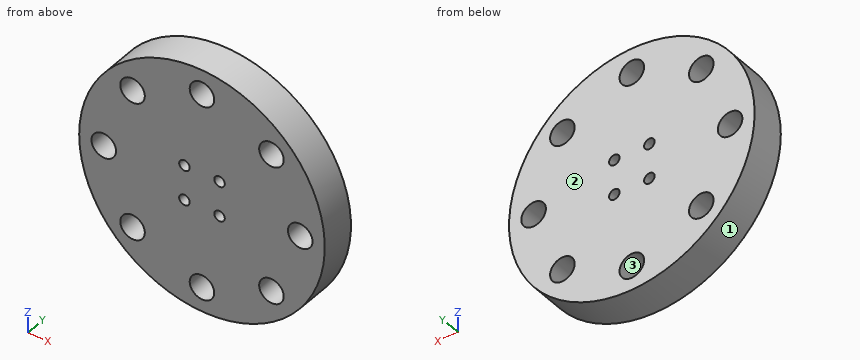
Autodesk Inventor part; units mm, degrees
ref_plane "YZ Plane" through (0, 0, 0) normal (1, 0, 0) x (0, 1, 0)
ref_plane "XZ Plane" through (0, 0, 0) normal (0, 1, 0) x (-1, 0, 0)
ref_plane "XY Plane" through (0, 0, 0) normal (0, 0, 1) x (1, 0, 0)
sketch "Szkic1" plane through (0, 0, 0) normal (0, 1, 0) x (-1, 0, 0)
  circle A0 centre (0, 0) radius 10
  circle A1 centre (0, 0) radius 17.5
  line L0 (0, 17.5) -> (0, -17.5)
  line L1 (-17.5, 0) -> (17.5, 0)
  circle A2 centre (2.5, 2.5) radius 0.75
  circle A3 centre (2.5, -2.5) radius 0.75
  circle A4 centre (-2.5, 2.5) radius 0.75
  circle A5 centre (-2.5, -2.5) radius 0.75
  circle A6 centre (0, 14) radius 1.75
  circle A7 centre (0, -14) radius 1.75
  circle A8 centre (14, 0) radius 1.75
  circle A9 centre (-14, 0) radius 1.75
  line L2 (-2.5, -2.5) -> (-12.3744, -12.3744)
  line L3 (2.5, 2.5) -> (12.3744, 12.3744)
  line L4 (2.5, -2.5) -> (12.3744, -12.3744)
  line L5 (-2.5, 2.5) -> (-12.3744, 12.3744)
  circle A10 centre (9.8995, 9.8995) radius 1.75
  circle A11 centre (-9.8995, -9.8995) radius 1.75
  line L6 (-2.5, 2.5) -> (2.5, -2.5)
  line L7 (2.5, 2.5) -> (-2.5, -2.5)
  circle A12 centre (-9.8995, 9.8995) radius 1.75
  circle A13 centre (9.8995, -9.8995) radius 1.75
  dimension "d1" = 35
  dimension "d0" = 20
  dimension "d2" = 1.5
  dimension "d3" = 5
  dimension "d4" = 5
  dimension "d5" = 28
  dimension "d6" = 3.5
  dimension "d7" = 28
  dimension "d8" = 3.5
  dimension "d9" = 3.5
  dimension "d11" = 19.799
extrude "Wyciągnięcie proste1" add sketch "Szkic1" along normal blind 5 contours L1 L7 A2 L3 A0 | L1 A8 A1 L4 A13 A0 | A0 L4 A3 L6 L1 | A0 L3 A10 A1 L1 A8 | L3 A2 L7 L0 A0 | A0 L0 A6 A1 L3 A10 | L4 A13 A1 L0 A7 A0 | A0 L0 L6 A3 L4 | L6 A4 L5 A0 L0 | L7 A5 L2 A0 L1 | L1 A0 L5 A4 L6 | L0 A0 L2 A5 L7 | A0 L5 A12 A1 L0 A6 | L0 A7 A1 L2 A11 A0 | L1 A9 A1 L5 A12 A0 | A0 L2 A11 A1 L1 A9
properties part number "Forma-kolo_dol"
Can you work these out from the model? Positions are in its coordinate system, mm. Face numbers are marked on the shaded views. Give positions to 0.01 mm unless a question says otherwise; leave off trailing zeros. Loops run counter-clockwise (first coordinate to the right, second up) from the corner with the lowest first, then second, coordinate; pieces in that order, holes last. Notation, with made-up numbers: (57.25, 82) - (99.25, 82) arc R18 cw to (99.25, 90) - close; hole circle Ø3 at (18.25, -1.5). An arc over 180 degrees is marked (long way). Return JSON: item names as keys, results as strings.
1. I want a section at C-C on x = 2.5. Please give me the cut outline in (y, z), and give its area (3 significant figures).
Output values:
{"outline": "(0, -17.32) - (5, -17.32) - (5, -3.25) - (0, -3.25) - close; (0, -1.75) - (5, -1.75) - (5, 1.75) - (0, 1.75) - close; (0, 3.25) - (5, 3.25) - (5, 17.32) - (0, 17.32) - close", "area": "158 mm²"}
2. I want a section at D-D on y = 3.35. Give the number of separate pieces and of enclosed holes in the cut face, and give its area (3 significant figures).
Output values:
{"separate pieces": "1", "enclosed holes": "12", "area": "878 mm²"}
3. If I drill on line 1 (Z direction, x = 0, y = 0.4); line 2 (X direction, y = 2.05, z = 2.5), over which ranges is the centre line in solid material (lowest first)?
Output values:
{"line 1": "z = -17.5 to -15.75, -12.25 to 12.25, 15.75 to 17.5", "line 2": "x = -17.32 to -3.25, -1.75 to 1.75, 3.25 to 17.32"}
4. I'm going to push flat-ended pins straight in: pin 1 Ø5.5 at (x, z) = (-9.9, 9.9) entering from +Y; pin 2 Ø3 at (x, y) = (-7.5, 1.5) entering from +Z. Where does each tip first touch, or does it pass through?
Output values:
{"pin 1": "stops at y = 5", "pin 2": "stops at z = 16.44"}
5. I want a section at B-B on z = 0. Please give me the cut outline in (x, y), and give its area (3 significant figures).
Output values:
{"outline": "(-17.5, 0) - (-15.75, 0) - (-15.75, 5) - (-17.5, 5) - close; (-12.25, 0) - (12.25, 0) - (12.25, 5) - (-12.25, 5) - close; (15.75, 0) - (17.5, 0) - (17.5, 5) - (15.75, 5) - close", "area": "140 mm²"}
6. I want a section at A-A on x = -14. Please give me the cut outline in (y, z), and give its area (3 significant figures).
Output values:
{"outline": "(0, -10.5) - (5, -10.5) - (5, -1.75) - (0, -1.75) - close; (0, 1.75) - (5, 1.75) - (5, 10.5) - (0, 10.5) - close", "area": "87.5 mm²"}
7. We'd pull the mould along X, two halves only. Please class the marked faces 1, 2 and 3: +X half, -X half, draft (parallel to the pull), parting line (faces both ways), or undercut.
Output values:
{"face 1": "parting line", "face 2": "draft", "face 3": "undercut"}
